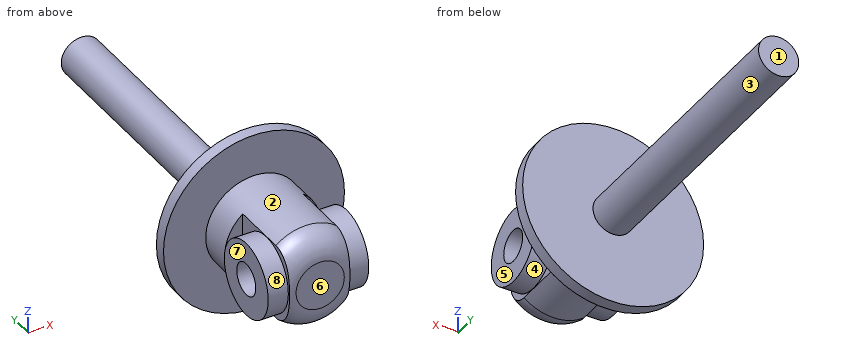
from build123d import *

# Parameters (mm, degrees)
SKETCH1_R               = 22.5
BOSS_EXTRUDE3_DEPTH     = 3
SKETCH3_R               = 5
BOSS_EXTRUDE4_DEPTH     = 70
SKETCH4_R               = 12
BOSS_EXTRUDE5_DEPTH     = 28
FILLET1_R               = 6
SKETCH6_W               = 20
SKETCH6_H               = 20
CUT_EXTRUDE1_DEPTH      = 23.5
CUT_EXTRUDE1_DEPTH_BACK = 23.5
SKETCH7_R               = 4
CUT_EXTRUDE2_DEPTH      = 28
SKETCH10_R              = 9.27822292
SKETCH10_R_2            = 4
BOSS_EXTRUDE6_DEPTH     = 12.5


with BuildPart() as part:
    # Sketch1 → Boss-Extrude3 (new body)
    with BuildSketch(Plane(origin=(0, 0, 0), x_dir=(1, 0, 0), z_dir=(0, 1, 0))):
        Circle(SKETCH1_R)
    extrude(amount=BOSS_EXTRUDE3_DEPTH)

    # Sketch3 → Boss-Extrude4 (add)
    with BuildSketch(Plane(origin=(0, 3, 0), x_dir=(1, 0, 0), z_dir=(0, 1, 0))):
        Circle(SKETCH3_R)
    extrude(amount=BOSS_EXTRUDE4_DEPTH)

    # Sketch4 → Boss-Extrude5 (add)
    with BuildSketch(Plane.XZ):
        Circle(SKETCH4_R)
    extrude(amount=BOSS_EXTRUDE5_DEPTH)

    # Fillet1
    fillet1_edges = [part.edges().sort_by_distance(p)[0] for p in [
        (-12, -28, 0),
    ]]
    fillet(fillet1_edges, radius=FILLET1_R)

    # Sketch6 → Cut-Extrude1 (cut, two sides)
    with BuildSketch(Plane.XY) as cut_extrude1_sk:
        with Locations((17.5, -18)):
            Rectangle(SKETCH6_W, SKETCH6_H)
        with Locations((-17.5, -18)):
            Rectangle(SKETCH6_W, SKETCH6_H)
    extrude(amount=CUT_EXTRUDE1_DEPTH, mode=Mode.SUBTRACT)
    extrude(cut_extrude1_sk.sketch, amount=-CUT_EXTRUDE1_DEPTH_BACK, mode=Mode.SUBTRACT)

    # Sketch7 → Cut-Extrude2 (cut)
    with BuildSketch(Plane(origin=(7.5, 0, 0), x_dir=(0, 0, -1), z_dir=(1, 0, 0))):
        with Locations((0, -18)):
            Circle(SKETCH7_R)
    extrude(amount=-CUT_EXTRUDE2_DEPTH, mode=Mode.SUBTRACT)

    # Sketch10 → Boss-Extrude6 (add, symmetric)
    with BuildSketch(Plane(origin=(0, 0, 0), x_dir=(0, 0, -1), z_dir=(1, 0, 0))):
        with Locations((0, -18)):
            Circle(SKETCH10_R)
        with Locations((0, -18)):
            Circle(SKETCH10_R_2, mode=Mode.SUBTRACT)
    extrude(amount=BOSS_EXTRUDE6_DEPTH, both=True)


solid = part.part
Build history of the part. All positions in model axes, mm. Face numbers are marked on the shaded views. A direction names the side the tool comes from. Round coordinates to 2 decimals unless told otherwise and drop trailing zeros. Write each loop counter-clockwise with the first axis right and the second up, starting at its lowest first coordinate (ties: lowest second). Pieces come first, ordered by that corner, then holes. Notation, with made-up numbers: (85, -7) - (102, -7) arc R9 ccw to (102, 10) - close; hole circle Ø11 at (59, 34). An arc over 180 degrees is marked (long way). Use CSV: the item, a comma, the result in double quotes.
(1) Pin check, flat tips, straight feed: P1, Ø8, axis at x = 6.5, y = 49.5, coming from the -Z side; P2, Ø5, axis at y = 14, z = -1.5, coming from the -X side; P3, Ø6, axis at y = 32.5, z = 6.5, coming from the -X side. Stop position of each tip, or through.
Response:
P1,"z = -4.33"
P2,"x = -5"
P3,"x = -3.57"
(2) Band-saw the part on B-B (x = -11). Write the cut outline in (y, z).
Response:
outline,"circle Ø18.56 at (-18, 0); (-8, -4.8) - (0, -4.8) - (0, -19.63) - (3, -19.63) - (3, 19.63) - (0, 19.63) - (0, 4.8) - (-8, 4.8) - close; hole circle Ø8 at (-18, 0)"
(3) Mould opens along Y. For the marked faces 1, 2 and 3 say: pulls with the +Y half, pulls with the -Y half, needs draft (parallel to the pull), parting line crosses it, or undercut.
Response:
face 1,"pulls with the +Y half"
face 2,"undercut"
face 3,"needs draft"
(4) Band-saw the part on D-D (z = -15). Write the cut outline in (x, y).
Response:
outline,"(-16.77, 0) - (16.77, 0) - (16.77, 3) - (-16.77, 3) - close"
(5) Wall check: line 1 (Y direction, x = 0, z = 0); line 2 (X direction, y = 17, z = 0); line 3 (Y direction, x = 17, z = 9.5). Give the ranges that are in metal, low to high.
Response:
line 1,"-28 to -22, -14 to 73"
line 2,"-5 to 5"
line 3,"0 to 3"
(6) Band-saw the part on C-C (y = 30). Write the cut outline in (x, z).
Response:
outline,"circle Ø10 at (0, 0)"
(7) Band-saw the part on A-A (y = -18). Write the cut outline in (x, z), plus the area to 3 significant figures.
Response:
outline,"(-12.5, -9.28) - (-7.5, -9.28) - (-7.5, -9.37) arc R12 ccw to (7.5, -9.37) - (7.5, -9.28) - (12.5, -9.28) - (12.5, -4) - (-12.5, -4) - close; (-12.5, 4) - (12.5, 4) - (12.5, 9.28) - (7.5, 9.28) - (7.5, 9.37) arc R12 ccw to (-7.5, 9.37) - (-7.5, 9.28) - (-12.5, 9.28) - close"
area,"321 mm²"
(8) 3-axis set-ups, long thin cutter, end or side, ignore diameter. For the marked faces 4, 5, 6, 7 and 8: which of +Z, -Z, +X, -X, +Y, -Y reach the whole face in a straight line?
Response:
face 4,"+X"
face 5,"+Z, -Z, +X, -Y"
face 6,"+Z, -Z, +X, -X, -Y"
face 7,"+Z, -Z, -X, -Y"
face 8,"-X"
